Autodesk Inventor part; units mm, degrees
ref_plane "Work Plane1" through (1.525, 0, 0) normal (0, 0, 1) x (1, 0, 0)
ref_plane "YZ Plane" through (0, 0, 0) normal (1, 0, 0) x (0, 1, 0)
ref_plane "XZ Plane" through (0, 0, 0) normal (0, 1, 0) x (-1, 0, 0)
sketch "Sketch1" plane through (0, 0, 0) normal (0, 0, 1) x (1, 0, 0)
  line L0 (0, 6.5) -> (0, 4)
  line L1 (3.7, 4) -> (80, 4)
  line L2 (80, 4) -> (80, 0)
  line L3 (80, 0) -> (-0.6001, 0)
  line L4 (-16.7201, 0) -> (96.12, 0)
  line L5 (-0.6001, 0) -> (-0.6001, 6.5)
  line L6 (-0.6001, 6.5) -> (0, 6.5)
  line L7 (3.7, 4) -> (2.9331, 4)
  line L8 (2.9331, 4) -> (0, 4)
  line L9 (0, -1.3) -> (0, 7.8)
  dimension "d0" = 80
  dimension "d1" = 76.3
  dimension "d2" = 8
  dimension "d9" = 0.6001
  dimension "d10" = 13
  dimension "d13" = 0.7669
  dimension "d14" = 8
revolve "Body" add sketch "Sketch1" angle 360 about axis through (80, 0, 0) along (-1, 0, 0)
sketch "Sketch2" plane through (-0.6001, 0, 0) normal (-1, 0, 0) x (0, 0, 1)
  line L0 (0, 7.5056) -> (6.5, 3.7528)
  line L1 (6.5, 3.7528) -> (6.5, -3.7528)
  line L2 (6.5, -3.7528) -> (0, -7.5056)
  line L3 (0, -7.5056) -> (-6.5, -3.7528)
  line L4 (-6.5, -3.7528) -> (-6.5, 3.7528)
  line L5 (-6.5, 3.7528) -> (0, 7.5056)
  point P0 (0, 0)
  point P1 (0, 0)
  dimension "d11" = 13
extrude "Head" add sketch "Sketch2" along normal blind 4.7
sketch "Sketch4" plane through (0, 0, 0) normal (0, 0, 1) x (1, 0, 0)
  line L0 (-5.3001, 6.5) -> (-5.3001, 7.5056)
  line L1 (-5.3001, 7.5056) -> (-4.7195, 7.5056)
  line L2 (-4.7195, 7.5056) -> (-5.3001, 6.5)
  line L3 (-6.2401, 0) -> (0.3399, 0)
  line L4 (-0.6001, 7.5056) -> (-5.3001, 7.5056)
  line L5 (-5.3001, 3.7528) -> (-5.3001, 7.5056)
  dimension "d5" = 30
  dimension "d19" = 13
revolve "Chamfer1" cut sketch "Sketch4" angle 360 about axis through (-10, 0, 0) along (1, 0, 0)
thread "Thread"
chamfer "Chamfer2" distance 0.7668 distance2 0.7669 1 edges at (80, -4, 0) measured on face at (80, -0.998, -0.8842)
ref_plane "Work Plane1" through (1.525, 0, 0) normal (0, 0, 1) x (1, 0, 0)
equation "\"d0\" = NLG"
equation "\"d1\" = GEL"
equation "\"d2\" = GD"
equation "\"d10\" = SD2"
equation "\"d14\" = BDM"
equation "\"d11\" = SW"
equation "\"d3\" = KOH - SD"
equation "\"d5\" = ANG1"
equation "\"d19\" = SW0"
equation "\"d15\" = GEL"
equation "\"d6\" = -0.5 * SPD + 0.5 * GD"
equation "\"NLG\" = 80"
equation "\"GD\" = NND"
equation "\"BDM\" = NND"
equation "\"KOH\" = 5.3"
equation "\"GEL\" = 76.3"
equation "\"SW\" = 13"
equation "\"SW0\" = SW"
equation "\"SPD\" = NND - 1.2269 * PTC"
equation "\"SD2\" = SW"
equation "\"SD\" = 0.6"
equation "\"ANG1\" = 30deg"
equation "\"GAL\" = 0.61345 * PTC"
equation "\"GUL\" = 0.61345 * PTC"
equation "\"RR\" = 0.4"
equation "\"WFT\" = SD"
equation "\"GD1\" = THREADDIA - 1.2269 * PTC"
equation "\"THREADDIA\" = 8"
equation "\"SDH\" = SW"
equation "\"TOA\" = 30deg"
equation "\"FAWI\" = 45deg"
equation "\"PTC\" = 1.25"
equation "\"NND\" = 8"
equation "\"E0\" = 1.155 * SW"
properties part number "AS 1110 - M8 x 80" material "Steel, Mild"
Work out the finished part from the listing and answer in its coordinate system (mm). A direction names the side the tool comes from. Coordinates: 2 decimals unless noted, no trailing zeros. Write each loop counter-clockwise with the first axis right and the second up, starting at its lowest first coordinate (ties: lowest second). Pieces come first, ordered by that corner, then holes. Notation, with made-up numbers: M 11,-29.75 L 33,-29.75 A27 cw 33,-1.75 Z; hole C 27.25,-8.5 d7. An arc over 180 degrees is marked long. Write item = value, one per line.
1. Flat-ended cylindrical pins translate along their axes: pin 1 (2 mm diameter, centred on x = 70.5, z = 4.5, fed in from +Y); pin 2 (5 mm diameter, centred on y = -5.5, z = 4, fed in from +X); pin 3 (2 mm diameter, centred on x = 55, z = -1.5, fed in from +Y). Find the tip coordinate at first contact, or state that the pin passes through.
Solution:
pin_1 = 1.94
pin_2 = 0
pin_3 = 3.97
2. Straight lines are drawn through the part: line 1 (X direction, y = -5, z = 1.5); line 2 (Z direction, x = 15.5, y = -0.75); line 3 (Z direction, x = 47.5, y = -1.75). For each, find the intervals that lie inside material, in ascending order. Write a range as from..to.
Solution:
line_1 = -5.3..0
line_2 = -3.93..3.93
line_3 = -3.6..3.6
3. For faces 1 (the face through (-0.6, 7, 0)), 2 (the face through (-0.6, -7, 0)), 3 (the face through (-0.296, -5.158, -3.955)), determine the directions among +Z, -Z, +X, -X, +Y, -Y from which every point of the face is accessible in a straight line to the end or side of a thin tool.
Solution:
face_1 = +X, +Y
face_2 = +X, -Y
face_3 = +X
4. The part is cut by section A-A (x = 34.5). Determine the outline of the cut face in (y, z), then the cut area to 3 significant figures.
Solution:
outline = C 0,0 d8
area = 50.3 mm2
